The figure shows three views and two pictorial views of one solid part (mm, origin at its lowest corner). Answer the questions. A direction names the side the tool comes from. Round coordinates to 2 decimals unless told otherwise and drop trailing zeros. Order: outer loops, then holes, each group sorted by start corner. A loop starts at its lowest first (then second) coordinate and runs counter-clockwise, first axis right, second up. Notation, with made-up numbers: (14, 45.25) - (37, 45.25) arc R31 ccw to (37, 70.25) - close; hole circle Ø7 at (89.5, 51). An arc over 180 degrees is marked (long way). Write item = value, one per line.
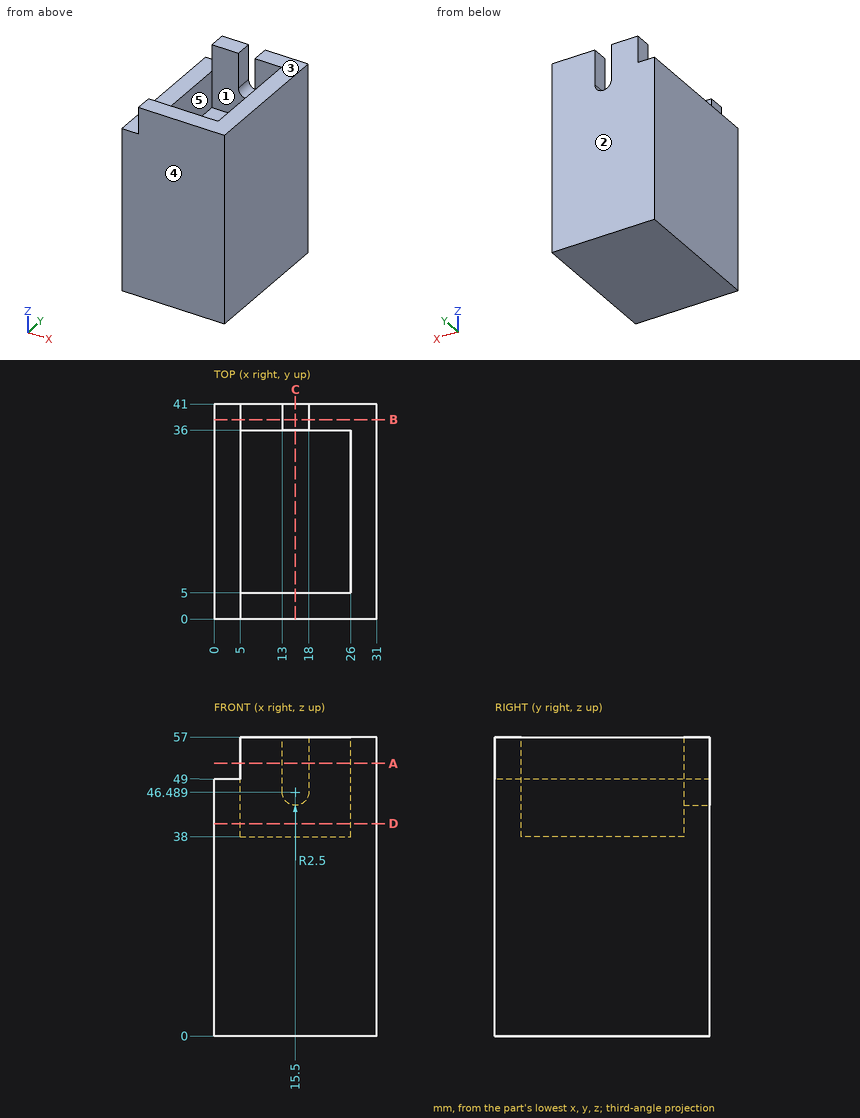
Q1. Flat-ended cylindrical pins translate along their axes: P1, Ø2.5, axis at x = 1.5, y = 22, coming from the +Z side; P2, Ø17, axis at x = 15, y = 22, coming from the +Z side; P3, Ø2.5, axis at y = 37.5, z = 52, coming from the -X side. Find the tip coordinate at first contact, or state that the pin passes through.
Model answer:
P1 = 49
P2 = 38
P3 = 5
Q2. Section C-C on x = 15.5 is taken. Determine the outline of the cut face in (y, z).
Model answer:
outline = (0, 0) - (41, 0) - (41, 43.99) - (36, 43.99) - (36, 38) - (5, 38) - (5, 57) - (0, 57) - close
Q3. For the marked faces 1 and 2, determine the directions among +Z, -Z, +X, -X, +Y, -Y from which every point of the face is accessible in a straight line to the end or side of a thin tool.
Model answer:
face_1 = +Z
face_2 = +Z, -Z, +X, -X, +Y
Q4. Section A-A on z = 52 is taken. Determine the outline of the cut face in (x, y).
Model answer:
outline = (5, 0) - (31, 0) - (31, 41) - (18, 41) - (18, 36) - (26, 36) - (26, 5) - (5, 5) - close; (5, 36) - (13, 36) - (13, 41) - (5, 41) - close
Q5. Section B-B on y = 38 is taken. Determine the outline of the cut face in (x, z).
Model answer:
outline = (0, 0) - (31, 0) - (31, 57) - (18, 57) - (18, 46.49) arc R2.5 cw to (13, 46.49) - (13, 57) - (5, 57) - (5, 49) - (0, 49) - close
Q6. Find the intervals of material crossed by line 1 (X direction, y = 9, z = 40); line 2 (X direction, y = 39.5, z = 46.5); line 3 (Y direction, x = 16.5, z = 41), in increasing order. Write a range as from..to.
Model answer:
line_1 = 0..5, 26..31
line_2 = 0..13, 18..31
line_3 = 0..5, 36..41
Q7. Determine the mould class of the marked faces 3, 4 and 5 for opening direction Y: released by +Y, released by -Y, zero draft, split by the parting line, or undercut.
Model answer:
face_3 = zero draft
face_4 = released by -Y
face_5 = undercut
Q8. Section D-D on z = 40.5 is taken. Determine the outline of the cut face in (x, y).
Model answer:
outline = (0, 0) - (31, 0) - (31, 41) - (0, 41) - close; hole (5, 5) - (26, 5) - (26, 36) - (5, 36) - close
